```python
from build123d import *
from build123d.topology import SkipClean

# Parameters (mm, degrees)
SKETCH1_W                    = 100
SKETCH1_H                    = 30
BASE_FLANGE1_DEPTH           = 3
EDGE_FLANGE1_STRIP_W         = 22
EDGE_FLANGE1_STRIP_H         = 3
EDGE_FLANGE1_STRIP_CUT_DEPTH = 100
EDGE_FLANGE1_DEPTH           = 100
EDGE_FLANGE2_DEPTH           = 97
EDGE_FLANGE2_START           = 3
EDGE_FLANGE2_FLAT_DEPTH      = 3
EDGE_FLANGE3_DEPTH           = 50
SKETCH16_R                   = 6
CUT_EXTRUDE1_DEPTH           = 10
SKETCH17_R                   = 41
CUT_EXTRUDE2_DEPTH           = 10
FILLET1_R                    = 7


# Sheet-metal steps are written as plain solids
with BuildPart() as part:
    # Sketch1 → Base-Flange1 (new body)
    with BuildSketch(Plane(origin=(0, 0, 0), x_dir=(0, 1, 0), z_dir=(0, 0, 1))):
        Rectangle(SKETCH1_W, SKETCH1_H)
    extrude(amount=BASE_FLANGE1_DEPTH)

    # Edge-Flange1 strip (across the edge) → Edge-Flange1 strip cut (cut)
    with BuildSketch(Plane(origin=(-15, 50, 3), x_dir=(1, 0, 0), z_dir=(0, -1, 0))):
        with Locations((-3, -1.5)):
            Rectangle(EDGE_FLANGE1_STRIP_W, EDGE_FLANGE1_STRIP_H)
    extrude(amount=EDGE_FLANGE1_STRIP_CUT_DEPTH, mode=Mode.SUBTRACT)

    # Edge-Flange1 section (across the edge) → Edge-Flange1 (add)
    with BuildSketch(Plane(origin=(-15, 50, 3), x_dir=(1, 0, 0), z_dir=(0, -1, 0))):
        with BuildLine():
            Line((0, 5), (0, 102))
            Line((0, 102), (3, 102))
            Line((3, 102), (3, 5))
            ThreePointArc((3, 5), (4.464466094, 1.464466094), (8, 0))
            Line((8, 0), (8, -3))
            ThreePointArc((8, -3), (2.343145751, -0.656854249), (0, 5))
        make_face()
    extrude(amount=EDGE_FLANGE1_DEPTH)

    # Edge-Flange2 bend section (across the edge) → Edge-Flange2 (add)
    with BuildSketch(Plane(origin=(-12, 55, 8), x_dir=(0, -1, 0), z_dir=(0, 0, 1))):
        with BuildLine():
            Line((-3, 5), (0, 5))
            ThreePointArc((0, 5), (1.464466094, 1.464466094), (5, 0))
            Line((5, 0), (5, -3))
            ThreePointArc((5, -3), (-0.656854249, -0.656854249), (-3, 5))
        make_face()
    extrude(amount=EDGE_FLANGE2_DEPTH)

    # Edge-Flange2 profile (on flange) → Edge-Flange2 flat (add)
    with BuildSketch(Plane(origin=(-12, 55, 0), x_dir=(0, 0, 1), z_dir=(0, 1, 0)).offset(EDGE_FLANGE2_START)):
        with BuildLine():
            Line((8, 5), (105, 5))
            Line((105, 5), (105, 9))
            Line((105, 9), (47.688860651, 85.054450695))
            ThreePointArc((47.688860651, 85.054450695), (37.115729743, 93.848030848), (23.729795349, 97))
            Line((23.729795349, 97), (8, 97))
            Line((8, 97), (8, 5))
        make_face()
    extrude(amount=-EDGE_FLANGE2_FLAT_DEPTH)

    # Edge-Flange3 section (across the edge) → Edge-Flange3 (add)
    with BuildSketch(Plane(origin=(35, 55, 3), x_dir=(0, 0, 1), z_dir=(1, 0, 0))):
        with BuildLine():
            Line((-3, 5), (-3, 32))
            Line((-3, 32), (0, 32))
            Line((0, 32), (0, 5))
            ThreePointArc((0, 5), (1.464466094, 1.464466094), (5, 0))
            Line((5, 0), (5, -3))
            ThreePointArc((5, -3), (-0.656854249, -0.656854249), (-3, 5))
        make_face()
    extrude(amount=EDGE_FLANGE3_DEPTH)

    # Sketch16 → Cut-Extrude1 (cut)
    with BuildSketch(Plane.XY.offset(3)):
        with Locations((60, 35)):
            Circle(SKETCH16_R)
    extrude(amount=-CUT_EXTRUDE1_DEPTH, mode=Mode.SUBTRACT)

    # Sketch17 → Cut-Extrude2 (cut)
    with BuildSketch(Plane(origin=(-15, 0, 0), x_dir=(0, -1, 0), z_dir=(-1, 0, 0))):
        with Locations(Location((0, 55, 0), (0, 0, 90))):
            Circle(SKETCH17_R)
    extrude(amount=-CUT_EXTRUDE2_DEPTH, mode=Mode.SUBTRACT)

    # Fillet1
    fillet1_edges = [part.edges().sort_by_distance(p)[0] for p in [
        (15, 50, 1.5),
        (35, 23, 1.5),
        (85, 23, 1.5),
    ]]
    fillet(fillet1_edges, radius=FILLET1_R)

    # SurfaceCut1
    split(bisect_by=Plane(origin=(0, 0, 0), x_dir=(-1, 0, 0), z_dir=(0, 1, 0)), keep=Keep.TOP)

    # Mirror2: part across plane


with BuildPart() as part_1:
    with SkipClean():  # the faces are left unmerged after this step: merging them gives an invalid solid
        add(part.part)
        add(part.part.mirror(Plane.ZX))

    # SurfaceCut2
    split(bisect_by=Plane(origin=(0, 0, 0), x_dir=(-1, 0, 0), z_dir=(0, 1, 0)), keep=Keep.TOP)

    # Mirror3: part across plane


with BuildPart() as part_2:
    with SkipClean():  # the faces are left unmerged after this step: merging them gives an invalid solid
        add(part_1.part)
        add(part_1.part.mirror(Plane.ZX))


solid = part_2.part
```
Could you check a few things on this model? Use its own coordinates, in mm. A direction names the side the tool comes from. Round coordinates to 2 decimals unless told otherwise and drop trailing zeros. Loops run counter-clockwise (first coordinate to the right, second up) from the corner with the lowest first, then second, coordinate; pieces in that order, holes last.
Q1. I want a section at D-D (z = 80). Write out the boundary of the cut face in (x, y), and give its area (3 significant figures).
Q2. I want a section at B-B (z = 11). Write out the boundary of the cut face in (x, y).
Q3. Thinking about a two-plate mould opening in Y: for faces 4 (the flat face through (60, 42, 3)), 5 (the cylindrical face through (37, 25.1, 1.5)), 6 (the cylindrical face through (-12.719, 55.594, 55.821)), 7 (the flat face through (85, -49, 2)), which applies, pulls with the +Y half, pulls with the -Y half, needs draft (parallel to the pull), parting line crosses it, or undercut?
Q4. Please list where these lines run through material, in increasing order: L1, parallel to Y at x = 29.5, z = 18; L2, parallel to Y at x = 60, z = 1.55; L3, parallel to X at y = -35, z = 0.95.
Q5. I want a section at C-C (x = 51.5). Write out the boundary of the cut face in (y, z), and give its area (3 significant figures).
Q6. On a 3-axis mill with a long thin cutter (end or side, diameter ignored), from which of +Z, -Z, +X, -X, +Y, -Y can I reach the whole of each face in a straight line? I mean faces 1 (the flat face through (35, 44, 2)), 2 (the flat face through (-12, -23, 90)), 3 (the flat face through (60, 23, 1)). Say none if no direction works.
Q7. For P1, Ø12, axis at x = 3, y = -41, coming from the +Z side; P2, Ø4, axis at y = -44.5, z = 3, coming from the -X side; P3, Ø2.5, axis at x = 52, z = 1, coming from the -Y side, each with a flat end and sliding along its axis, tell me the tip position at first contact or that it passes through.
Q8. I want a section at A-A (y = 0). Write out the boundary of the cut face in (x, z).
Answer below:
1. outline: (-15, -50) arc R8 ccw to (-7, -58) - (30.18, -58) - (30.18, -55) - (-7, -55) arc R5 cw to (-12, -50) - (-12, -32.5) - (-15, -32.5) - close; (-15, 32.5) - (-12, 32.5) - (-12, 50) arc R5 cw to (-7, 55) - (30.18, 55) - (30.18, 58) - (-7, 58) arc R8 ccw to (-15, 50) - close
1. area: 389 mm2
2. outline: (-15, -50) arc R8 ccw to (-7, -58) - (85, -58) - (85, -55) - (-7, -55) arc R5 cw to (-12, -50) - (-12, 50) arc R5 cw to (-7, 55) - (85, 55) - (85, 58) - (-7, 58) arc R8 ccw to (-15, 50) - close
3. face 4: undercut
3. face 5: undercut
3. face 6: pulls with the +Y half
3. face 7: needs draft
4. L1: y = -58 to -55, 55 to 58
4. L2: y = -54.73 to -41, -29 to -23, 23 to 29, 41 to 54.73
4. L3: x = -10.78 to 15, 35 to 54, 66 to 85
5. outline: (-58, 8) arc R8 ccw to (-50, 0) - (-23, 0) - (-23, 3) - (-50, 3) arc R5 cw to (-55, 8) - (-55, 63.93) - (-58, 63.93) - close; (23, 0) - (50, 0) arc R8 ccw to (58, 8) - (58, 63.93) - (55, 63.93) - (55, 8) arc R5 cw to (50, 3) - (23, 3) - close
5. area: 559 mm2
6. face 1: -Z, +Y, -Y
6. face 2: +Z, +X
6. face 3: +Z, -Z, +X
7. P1: stops at z = 3
7. P2: stops at x = -14.42
7. P3: stops at y = -55.56
8. outline: (-15, 8) arc R8 ccw to (-7, 0) - (15, 0) - (15, 3) - (-7, 3) arc R5 cw to (-12, 8) - (-12, 14) - (-15, 14) - close; (-15, 96) - (-12, 96) - (-12, 105) - (-15, 105) - close
